Check sheet for the modelled part. Datum: model origin and axes. Units: mm. Face numbers are marked on the shaded views. A direction names the side the tool comes from. Round coordinates to 2 decimals unless told otherwise and drop trailing zeros. Write each loop counter-clockwise with the first axis right and the second up, starting at its lowest first coordinate (ties: lowest second). Pieces come first, ordered by that corner, then holes. Notation, with made-up numbers: (13, -5.75) -> (29, -5.75) arc R15 ccw to (29, 23.25) -> close; hole circle Ø6 at (58.5, -31). An arc over 180 degrees is marked (long way). Write item = value, one per line.
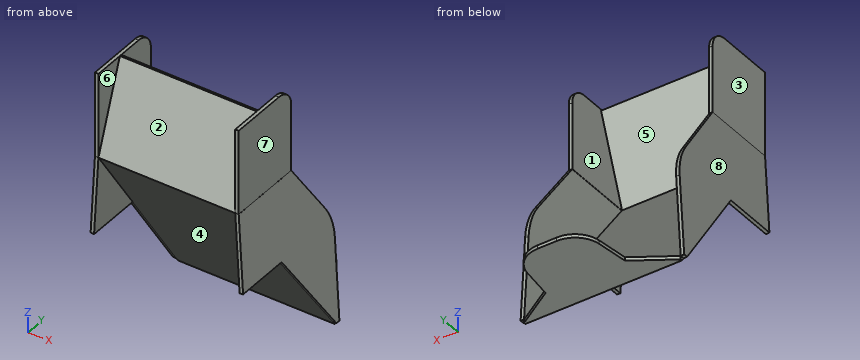
from build123d import *

# Parameters (mm, degrees)
BOSS_EXTRUDE1_DEPTH     = 450.85
CUT_EXTRUDE2_DEPTH      = 508
FILLET1_R               = 76.2
SKETCH8_W               = 28.575
SKETCH8_H               = 250.515691668
CUT_EXTRUDE3_DEPTH      = 244.471906543
CUT_EXTRUDE3_DEPTH_BACK = 361.52650092
BOSS_EXTRUDE4_DEPTH     = 10
SKETCH11_W              = 243.025134326
SKETCH11_H              = 216.946269836
BOSS_EXTRUDE5_DEPTH     = 10
FILLET2_R               = 177.8
FILLET3_R               = 50.8
FILLET2_OF_MIRROR1_R    = 177.8
FILLET3_OF_MIRROR1_R    = 50.8


with BuildPart() as part:
    # Sketch1 → Boss-Extrude1 (new body)
    with BuildSketch(Plane(origin=(0, 0, 0), x_dir=(0, 0, -1), z_dir=(1, 0, 0))):
        Polygon((-172.951120204, -349.34913054), (-411.633045884, -262.476014135), (-415.053247317, -271.872940343), (-171.479591477, -360.52650092), (357.210427919, 9.666236038), (357.210427919, 243.471906543), (347.210427919, 243.471906543), (347.210427919, 14.871906543), align=None)
    extrude(amount=BOSS_EXTRUDE1_DEPTH)

    # Sketch3 → Cut-Extrude2 (cut)
    with BuildSketch(Plane.XY.offset(-347.210427919)):
        Polygon((450.85, 243.471906543), (320.675, 243.471906543), (339.725, 85.650531553), (450.85, 14.871906543), align=None)
        Polygon((111.125, 85.650531553), (130.175, 243.471906543), (0, 243.471906543), (0, 14.871906543), align=None)
    extrude(amount=-CUT_EXTRUDE2_DEPTH, mode=Mode.SUBTRACT)

    # Fillet1
    fillet1_edges = [part.edges().sort_by_distance(p)[0] for p in [
        (320.675, 243.471906543, -352.210427919),
        (130.175, 243.471906543, -352.210427919),
    ]]
    fillet(fillet1_edges, radius=FILLET1_R)

    # Sketch8 → Cut-Extrude3 (cut, two sides)
    with BuildSketch(Plane(origin=(0, 0, 0), x_dir=(1, 0, 0), z_dir=(0, 1, 0))) as cut_extrude3_sk:
        Polygon((0, -172.951120204), (0, 347.210427919), (28.575, -172.951120204), align=None)
        Polygon((422.275, -172.951120204), (450.85, -172.951120204), (450.85, 347.210427919), align=None)
        with Locations((436.5625, -298.208966038)):
            Rectangle(SKETCH8_W, SKETCH8_H)
        with Locations((14.2875, -298.208966038)):
            Rectangle(SKETCH8_W, SKETCH8_H)
    extrude(amount=CUT_EXTRUDE3_DEPTH, mode=Mode.SUBTRACT)
    extrude(cut_extrude3_sk.sketch, amount=-CUT_EXTRUDE3_DEPTH_BACK, mode=Mode.SUBTRACT)

    # Sketch9 → Boss-Extrude4 (add)
    with BuildSketch(Plane(origin=(19.016566107, 0, -1.04467233), x_dir=(0.054852151, 0, 0.998494487), z_dir=(-0.998494487, 0, 0.054852151))):
        Polygon((-53.849912427, 14.871906543), (-346.687698266, 14.871906543), (172.784392877, -348.318755032), (172.784392877, -143.580231084), align=None)
        Polygon((172.784392877, -360.52650092), (-55.252957085, -201.093419897), (-55.252957085, -360.52650092), align=None)
        Polygon((172.784392877, -348.318755032), (-346.687698266, 14.871906543), (-346.687698266, 2.664160656), (-55.252957085, -201.093419897), (172.784392877, -360.52650092), align=None)
    boss_extrude4 = extrude(amount=BOSS_EXTRUDE4_DEPTH)

    # Sketch11 → Boss-Extrude5 (add)
    with BuildSketch(Plane.ZY.offset(-28.575)):
        with Locations((293.540680154, -252.053366002)):
            Rectangle(SKETCH11_W, SKETCH11_H)
    boss_extrude5 = extrude(amount=BOSS_EXTRUDE5_DEPTH)

    # Fillet2
    fillet2_edges = [part.edges().sort_by_distance(p)[0] for p in [
        (11.070310121, 14.871906543, -54.539252282),
    ]]
    fillet(fillet2_edges, radius=FILLET2_R)

    # Fillet3
    fillet3_edges = [part.edges().sort_by_distance(p)[0] for p in [
        (23.575, -143.580231084, 415.053247317),
    ]]
    fillet(fillet3_edges, radius=FILLET3_R)

    # Mirror1: Boss-Extrude4, Boss-Extrude5 across plane
    add(boss_extrude4.mirror(Plane(origin=(225.425, 0, 0), x_dir=(0, 0, 1), z_dir=(1, 0, 0))))
    add(boss_extrude5.mirror(Plane(origin=(225.425, 0, 0), x_dir=(0, 0, 1), z_dir=(1, 0, 0))))

    # Fillet2 of Mirror1
    fillet2_of_mirror1_edges = [part.edges().sort_by_distance(p)[0] for p in [
        (439.779689879, 14.871906543, -54.539252282),
    ]]
    fillet(fillet2_of_mirror1_edges, radius=FILLET2_OF_MIRROR1_R)

    # Fillet3 of Mirror1
    fillet3_of_mirror1_edges = [part.edges().sort_by_distance(p)[0] for p in [
        (427.275, -143.580231084, 415.053247317),
    ]]
    fillet(fillet3_of_mirror1_edges, radius=FILLET3_OF_MIRROR1_R)


solid = part.part
(1) Material ranges on L1, parallel to X at y = -299, z = 180.5 (3 decimals); L2, parallel to Z at x = 306.5, y = 106.5; L3, parallel to X at y = -312, z = 155, recorded low to high. Write a range as [from, to].
Worked answers:
L1 = [18.575, 28.575], [422.275, 432.275]
L2 = [-357.21, -347.21]
L3 = [17.57, 27.59], [423.26, 433.28]
(2) Sectioned sample at D-D on z = 277. Enter the section's corners in (x, y) (1 decimal), then the cut area to 3 significant figures.
Worked answers:
outline = (18.6, -360.5) -> (28.6, -360.5) -> (28.6, -322.1) -> (422.3, -322.1) -> (422.3, -360.5) -> (432.3, -360.5) -> (432.3, -143.6) -> (422.3, -143.6) -> (422.3, -311.5) -> (28.6, -311.5) -> (28.6, -143.6) -> (18.6, -143.6) -> close
area = 8,530 mm²
(3) Sectioned sample at B-B on x = 307. Enter the section's corners in (y, z), then the cut area to 3 significant figures.
Worked answers:
outline = (-360.53, 171.48) -> (9.67, -357.21) -> (221.15, -357.21) -> (221.15, -347.21) -> (14.87, -347.21) -> (-349.35, 172.95) -> (-262.48, 411.63) -> (-271.87, 415.05) -> close
area = 11,100 mm²
(4) Access from +Z, -Z, +X, -X, +Y, -Y to the whole of each face (thin tool, end or side, straight path). Record for the marked faces 4, 5, 6, 7 and 8.
Worked answers:
face_4 = -Z, -Y
face_5 = +Y
face_6 = +Z, -Y
face_7 = +Z, +X, +Y, -Y
face_8 = +Z, -X, +Y, -Y
(5) Sectioned sample at C-C on y = -314. Enter the section's corners in (x, z) (3 decimals), then the cut area to 3 significant figures.
Worked answers:
outline = (6.001, -55.666) -> (15.986, -56.214) -> (24.844, 105.033) -> (426.006, 105.033) -> (434.864, -56.214) -> (444.849, -55.666) -> (432.341, 172.028) -> (422.356, 171.48) -> (425.048, 122.467) -> (25.802, 122.467) -> (28.494, 171.48) -> (18.509, 172.028) -> close; (18.575, 172.028) -> (28.575, 172.028) -> (28.575, 270.072) -> (422.275, 270.072) -> (422.275, 172.028) -> (432.275, 172.028) -> (432.275, 415.053) -> (422.275, 415.053) -> (422.275, 299.31) -> (28.575, 299.31) -> (28.575, 415.053) -> (18.575, 415.053) -> close
area = 27,900 mm²
(6) Go/stop test with flat-tipped pins: P1, Ø5, axis at y = 6, z = -350, coming from the -X side; P2, Ø5, axis at x = 21.5, y = -220, coming from the -Z side; P3, Ø10, axis at y = -151.5, z = 151, coming from the +X side. Record where each tip stops, or that it passes through.
Worked answers:
P1 = 0
P2 = -32.78
P3 = 433.77
(7) Release check for a two-part mould opening along Z. For the marked faces 1, 2 and 3 record: pulls with the +Z half, pulls with the -Z half, needs draft (parallel to the pull), parting line crosses it, or undercut.
Worked answers:
face_1 = undercut
face_2 = pulls with the +Z half
face_3 = needs draft
(8) Sectioned sample at A-A on y = -128.5. Enter the section's corners in (x, z), then the cut area to 3 significant figures.
Worked answers:
outline = (0.31, -159.34) -> (10.29, -159.89) -> (440.56, -159.89) -> (450.54, -159.34) -> (433.52, 150.49) -> (423.54, 149.94) -> (439.6, -142.45) -> (11.25, -142.45) -> (27.31, 149.94) -> (17.33, 150.49) -> close
area = 13,700 mm²
